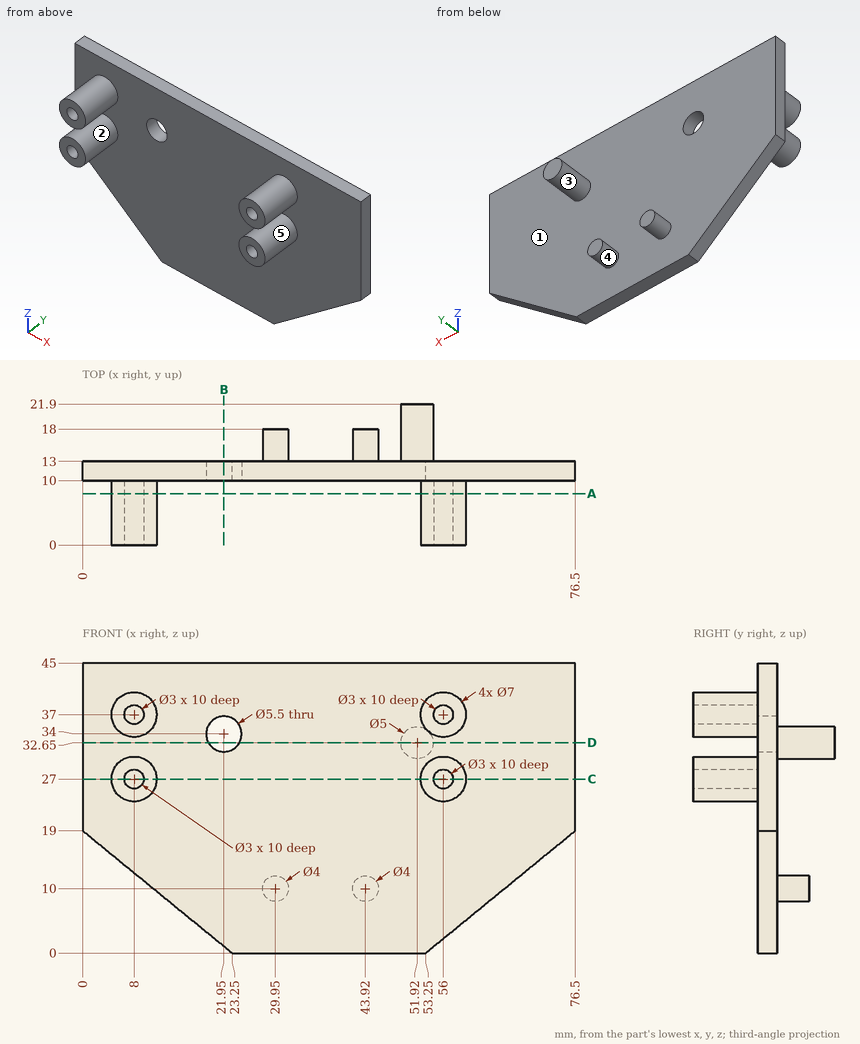
The figure shows three views and two pictorial views of one solid part (mm, origin at its lowest corner). Answer the questions. A direction names the side the tool comes from. Round coordinates to 2 decimals unless told otherwise and drop trailing zeros. Write each loop counter-clockwise with the first axis right and the second up, starting at its lowest first coordinate (ties: lowest second). Pieces come first, ordered by that corner, then holes. Notation, with made-up numbers: (4.5, -24) - (26.5, -24) arc R25 ccw to (26.5, -2) - close; hole circle Ø4 at (45.5, 37.5). An arc over 180 degrees is marked (long way). Answer in a Markdown table with one row per item. Add a question column.
1. A cutting plane is placed at D-D, the plane z = 32.65. Determine the outline of the cut face in (x, y).
2. Given pin 1 (2 mm diameter, centred on x = 44.5, z = 10.5, fed in from +Y); pin 2 (10 mm diameter, centred on y = 18.5, z = 14, fed in from -X); pin 3 (3.5 mm diameter, centred on x = 55.5, z = 27.5, fed in from -Y); pin 4 (1 mm diameter, centred on y = 12, z = 14.5, fed in from -X) (1 decimal), each flat-ended and moving along its own axis, determine where each tip first touches the part or whether it passes through.
3. A cutting plane is placed at C-C, the plane z = 27. Determine the outline of the cut face in (x, y).
4. A cutting plane is placed at A-A, the plane y = 8. Determine the outline of the cut face in (x, z), and give its area (3 significant figures).
5. For the marked faces 4 and 5, determine the directions among +Z, -Z, +X, -X, +Y, -Y from which every point of the face is accessible in a straight line to the end or side of a thin tool.
6. A cutting plane is placed at B-B, the plane x = 21.95. Determine the outline of the cut face in (y, z), and give its area (3 significant figures).
7. Find the intervals of material crossed by line 1 along X through (y, z) = (7.75, 37); line 2 along X through (y, z) = (5, 26) (1 decimal); line 3 along X through (y, z) = (10.7, 34), in increasing order. Write a range as from..to.
8. The mould has two halves that part along Z. Classify the marked faces 1, 2 and 3: +Z half, -Z half, draft (parallel to the pull), parting line (faces both ways), or undercut.
Worked out:
| question | item | result |
|---|---|---|
| 1 | outline | (0, 10) - (19.55, 10) - (19.55, 13) - (0, 13) - close; (24.35, 10) - (76.5, 10) - (76.5, 13) - (54.42, 13) - (54.42, 21.9) - (49.42, 21.9) - (49.42, 13) - (24.35, 13) - close |
| 2 | pin 1 | y = 18 |
| 2 | pin 2 | x = 27.95 |
| 2 | pin 3 | y = 0 |
| 2 | pin 4 | x = 4.9 |
| 3 | outline | (0, 10) - (4.5, 10) - (4.5, 0) - (6.5, 0) - (6.5, 10) - (9.5, 10) - (9.5, 0) - (11.5, 0) - (11.5, 10) - (52.5, 10) - (52.5, 0) - (54.5, 0) - (54.5, 10) - (57.5, 10) - (57.5, 0) - (59.5, 0) - (59.5, 10) - (76.5, 10) - (76.5, 13) - (0, 13) - close |
| 4 | outline | circle Ø7 at (8, 27); circle Ø7 at (8, 37); circle Ø7 at (56, 27); circle Ø7 at (56, 37); hole circle Ø3 at (8, 27); hole circle Ø3 at (8, 37); hole circle Ø3 at (56, 27); hole circle Ø3 at (56, 37) |
| 4 | area | 126 mm^2 |
| 5 | face 4 | +Y |
| 5 | face 5 | -Y |
| 6 | outline | (10, 1.06) - (13, 1.06) - (13, 31.25) - (10, 31.25) - close; (10, 36.75) - (13, 36.75) - (13, 45) - (10, 45) - close |
| 6 | area | 115 mm^2 |
| 7 | line 1 | 4.5..6.5, 9.5..11.5, 52.5..54.5, 57.5..59.5 |
| 7 | line 2 | 4.6..6.9, 9.1..11.4, 52.6..54.9, 57.1..59.4 |
| 7 | line 3 | 0..19.2, 24.7..76.5 |
| 8 | face 1 | draft |
| 8 | face 2 | undercut |
| 8 | face 3 | parting line |
